Check sheet for the drawn part. Datum: minimum x, y, z corner. Units: mm. Give positions to 0.01 mm unless a question says otherwise; leave off trailing zeros.
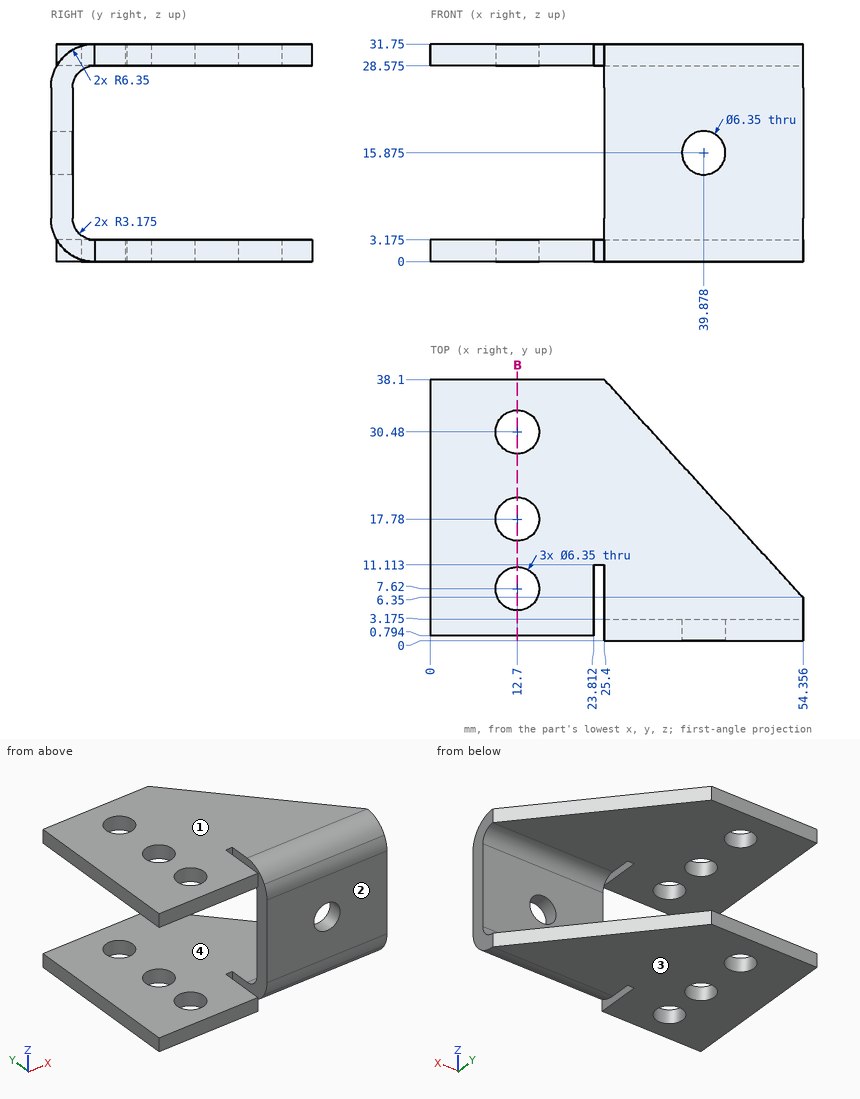
Item 1: Sectioned sample at B-B (x = 12.7). Give the number of separate pieces and of enclosed holes in the cut face, and give its area (3 significant figures).
Reported:
separate pieces: 8
enclosed holes: 0
area: 116 mm2
Item 2: Gauge pin test, flat ends, axial feed: pin 1 (3 mm diameter, centred on x = 47.5, z = 15, fed in from +Y) (1 decimal); pin 2 (1.7 mm diameter, centred on x = 24.5, z = 1, fed in from -Y); pin 3 (12 mm diameter, centred on y = 7.5, z = 15.5, fed in from -X). Record the tip position at first contact, or that the pin passes through.
Reported:
pin 1: stops at y = 3.2
pin 2: stops at y = 0.79
pin 3: stops at x = 25.4
Item 3: Scan lines: L1, parallel to Y at x = 12.7, z = 1.45 (1 decimal); L2, parallel to X at y = 7, z = 29 (1 decimal); L3, parallel to Y at x = 52, z = 12 (1 decimal). Record each from-to range of solid material in increasing order.
Reported:
L1: y = 0.8 to 4.4, 10.8 to 14.6, 21 to 27.3, 33.7 to 38.1
L2: x = 0 to 9.6, 15.8 to 23.8, 25.4 to 53.8
L3: y = 0 to 3.2
Item 4: Draft check along Z on the marked faces 1, 2, 3 and 4. Enter one of: released by +Z, released by -Z, zero draft, split by the parting line, or undercut.
Reported:
face 1: released by +Z
face 2: zero draft
face 3: released by -Z
face 4: undercut
